CAD build for the part. Positions are in the model's coordinates, mm. Give positions to 0.01 mm unless a question says otherwise; leave off trailing zeros. Loops run counter-clockwise (first coordinate to the right, second up) from the corner with the lowest first, then second, coordinate; pieces in that order, holes last. Notation, with made-up numbers: (35, 89) - (86, 89) arc R20 cw to (86, 124) - close; hole circle Ø2 at (51, 67.25). An arc over 180 degrees is marked (long way). Return JSON: item names as keys, results as strings.
from build123d import *

# Parameters (mm, degrees)
SKETCH2_W           = 10
SKETCH2_H           = 4.5
BOSS_EXTRUDE1_DEPTH = 4.5


with BuildPart() as part:
    # Sketch2 → Boss-Extrude1 (new body)
    with BuildSketch(Plane(origin=(0, 0, 0), x_dir=(1, 0, 0), z_dir=(0, 1, 0))):
        Polygon((11.295466324, 4.5), (11.295466324, 0), (-18.204533676, 0), (-18.204533676, -64), (-53.704533676, -64), (-53.704533676, 72), (-45.704533676, 72), (-45.704533676, 76.5), (38.295466324, 76.5), (38.295466324, 72), (59.995466324, 72), (59.995466324, 4.5), (56.995466324, 4.5), (56.995466324, 0), (59.995466324, 0), (59.995466324, -64), (26.295466324, -64), (26.295466324, -18.5), (39.295466324, -18.5), (39.295466324, -6), (26.295466324, -6), (26.295466324, 4.5), (16.295466324, 4.5), (16.295466324, 0), (14.295466324, 0), (14.295466324, 4.5), align=None)
        with Locations((49.995466324, 2.25)):
            Rectangle(SKETCH2_W, SKETCH2_H, mode=Mode.SUBTRACT)
        Polygon((-33.704533676, -15.5), (-33.704533676, -18.5), (-46.704533676, -18.5), (-46.704533676, -6), (-33.704533676, -6), (-33.704533676, -9), (-43.704533676, -9), (-43.704533676, -15.5), align=None, mode=Mode.SUBTRACT)
    extrude(amount=BOSS_EXTRUDE1_DEPTH)


solid = part.part
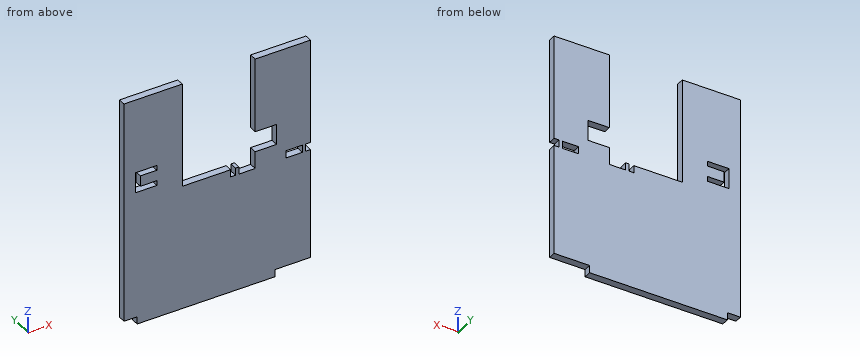
1. Drop flat-ended pins along their axis: P1, Ø1.3, axis at x = 49.5, y = 3, coming from the -Z side; P2, Ø1, axis at x = -11, y = 2, coming from the +Z side; P3, Ø1.3, axis at y = 3.5, z = -2, coming from the +X side. Give the stop position or say it passes through.
Values follow:
{"P1": "stops at z = -72", "P2": "stops at z = 0", "P3": "stops at x = 57"}
2. Cut at D-D, the plane x = 22. Write the cut outline in (y, z), plus the area to 3 significant figures.
Values follow:
{"outline": "(0, -76.5) - (4.5, -76.5) - (4.5, -4.5) - (0, -4.5) - close", "area": "324 mm²"}
3. Drill centre lines: probe 1 along Z at (x, y) = (-36, 0.2); probe 2 along X at (y, z) = (2.05, 17); probe 3 along X at (y, z) = (2.6, 56.5). Where is each one in solid material? Low to high.
Values follow:
{"probe 1": "z = -76.5 to 6, 9 to 15.5, 18.5 to 64", "probe 2": "x = -53.7 to -46.7, -33.7 to -18.2, 39.3 to 60", "probe 3": "x = -53.7 to -18.2, 26.3 to 60"}
4. Cut at A-A, the plane x = -38.5. Write the cut outline in (y, z), plus the area to 3 significant figures.
Values follow:
{"outline": "(0, -76.5) - (4.5, -76.5) - (4.5, 6) - (0, 6) - close; (0, 9) - (4.5, 9) - (4.5, 15.5) - (0, 15.5) - close; (0, 18.5) - (4.5, 18.5) - (4.5, 64) - (0, 64) - close", "area": "605 mm²"}
5. Cut at B-B, the plane z = -1.5. Write the cut outline in (x, y), plus the area to 3 significant figures.
Values follow:
{"outline": "(-53.7, 0) - (11.3, 0) - (11.3, 4.5) - (-53.7, 4.5) - close; (14.3, 0) - (16.3, 0) - (16.3, 4.5) - (14.3, 4.5) - close; (26.3, 0) - (45, 0) - (45, 4.5) - (26.3, 4.5) - close; (55, 0) - (57, 0) - (57, 4.5) - (55, 4.5) - close", "area": "395 mm²"}
6. Cut at C-C, the plane z = 26. Write the cut outline in (x, y).
Values follow:
{"outline": "(-53.7, 0) - (-18.2, 0) - (-18.2, 4.5) - (-53.7, 4.5) - close; (26.3, 0) - (60, 0) - (60, 4.5) - (26.3, 4.5) - close"}
